Design review of the part shown in the three views and the two pictorial views. Dimensions are in mm from the part's minimum x, y and z. A direction names the side the tool comes from. Round coordinates to 2 decimals unless told otherwise and drop trailing zeros. Write each loop counter-clockwise with the first axis right and the second up, starting at its lowest first coordinate (ties: lowest second). Pieces come first, ordered by that corner, then holes. Notation, with made-up numbers: (56, -21) -> (104, -21) arc R22 ccw to (104, -4) -> close; hole circle Ø11 at (-10, 82). An arc over 180 degrees is marked (long way). Return JSON: item names as keys, results as strings. Group by question number.
1. Tool access review of the marked faces 1 and 2: name each direction out of +Z, -Z, +X, -X, +Y, -Y from which nothing blocks a thin tool from reaching the whole face with its end or side.
2. Take a section at B-B, the plane x = 9. Write out the cut boundary in (y, z) (1 decimal), then the cut area to 3 significant figures.
3. Mouldability with a two-part tool opening along X and no side actions: class the marked faces 3, 4 and 5 as pulls with the +X half, pulls with the -X half, needs draft (parallel to the pull), parting line crosses it, or undercut.
4. For line 1 along X through (y, z) = (4.25, 9) (1 decimal); line 2 along Y through (x, z) = (10.25, 1.5), list the stretches that pass through material, from the lowest coordinate up. Write a range as from..to.
5. Take a section at A-A, the plane z = 9. Write out the cut boundary in (x, y) (1 decimal).
6. Take a section at D-D, the plane z = 3.5. Write out the cut boundary in (x, y), then the cut area to 3 significant figures.
7. Clearance check with flat-ended pins moving along their axes: P1, Ø9, axis at x = 12, z = 8, coming from the +Y side; P2, Ø1, axis at y = 1, z = 14.5, coming from the +X side. State where each tip first meets the part, or that it passes through.
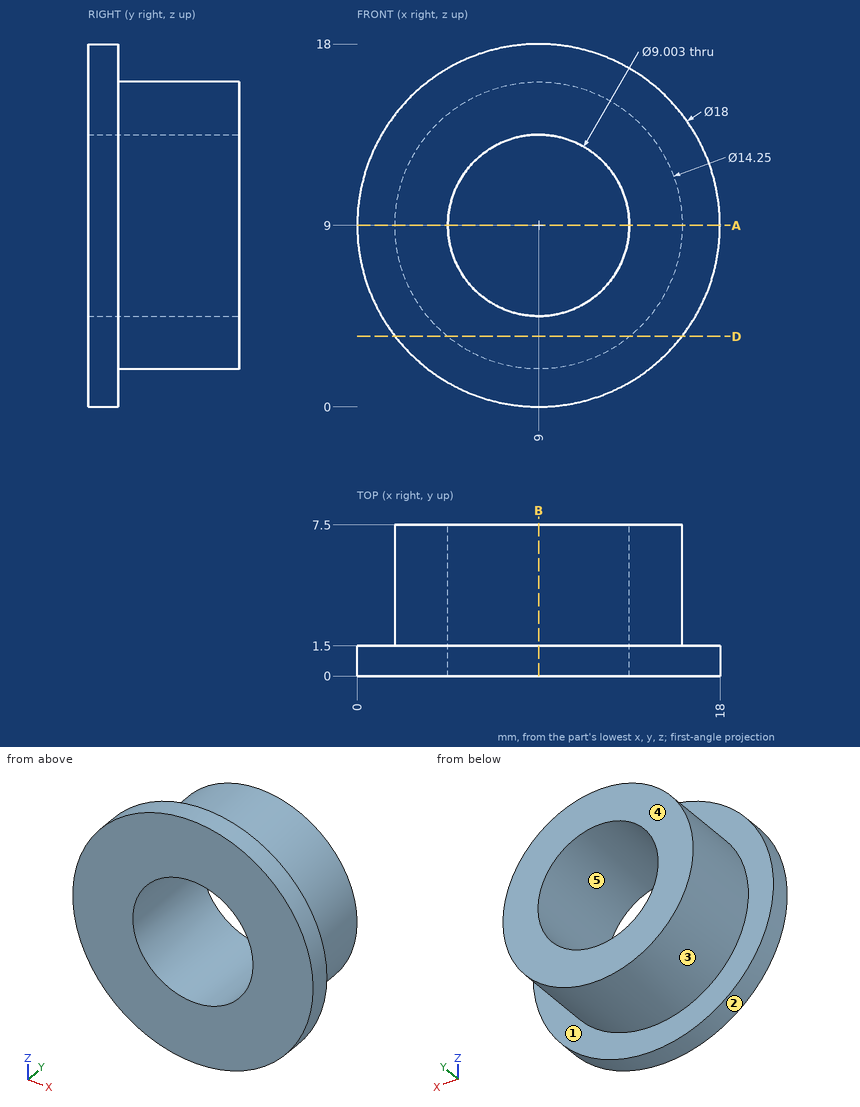
Output:
{
 "1": {"face 1": "+Y", "face 2": "+Y, -Y"},
 "2": {"outline": "(0, 0) -> (1.5, 0) -> (1.5, 1.9) -> (7.5, 1.9) -> (7.5, 4.5) -> (0, 4.5) -> close; (0, 13.5) -> (7.5, 13.5) -> (7.5, 16.1) -> (1.5, 16.1) -> (1.5, 18) -> (0, 18) -> close", "area": "45.0 mm^2"},
 "3": {"face 3": "parting line crosses it", "face 4": "needs draft", "face 5": "undercut"},
 "4": {"line 1": "x = 1.9..4.5, 13.5..16.1", "line 2": "y = 0..1.5"},
 "5": {"outline": "(0, 0) -> (4.5, 0) -> (4.5, 7.5) -> (1.9, 7.5) -> (1.9, 1.5) -> (0, 1.5) -> close; (13.5, 0) -> (18, 0) -> (18, 1.5) -> (16.1, 1.5) -> (16.1, 7.5) -> (13.5, 7.5) -> close"},
 "6": {"outline": "(1.88, 0) -> (16.12, 0) -> (16.12, 1.5) -> (13.53, 1.5) -> (13.53, 7.5) -> (4.47, 7.5) -> (4.47, 1.5) -> (1.88, 1.5) -> close", "area": "75.7 mm^2"},
 "7": {"P1": "stops at y = 7.5", "P2": "stops at x = 16.48"}
}
